The model under review builds one solid part; all positions refer to its coordinate system, in mm. A direction names the side the tool comes from. Coordinates: 2 decimals unless noted, no trailing zeros. Loops run counter-clockwise (first coordinate to the right, second up) from the corner with the lowest first, then second, coordinate; pieces in that order, holes last. Notation, with made-up numbers: (64, 12.25) - (103, 12.25) arc R23 ccw to (103, 46.25) - close; hole circle Ø6 at (12.25, 50.5). An arc over 180 degrees is marked (long way). One line per item, written item: value. Start each with the question number.
1. We need section C-C, the plane y = -8.25. Give the boundary of the cut face in (x, z).
2. We need section D-D, the plane x = -16. Give the boundary of the cut face in (y, z), then the cut area to 3 significant figures.
3. Insertion check: P1, Ø2, axis at y = -11.5, z = 36, coming from the -X side; P2, Ø6, axis at x = 3.5, y = 10, coming from the -Z side; P3, Ø9.5, axis at x = 23, z = 68.5, coming from the -Y side. Each pin has a flat end and moves straight along its axis. Give the tip position at first contact, or say it passes through.
4. For faces 5 (the face through (12.35, -12, 33)), 6 (the face through (21.34, -1.45, 64.78)), 7 (the face through (-25.8, 6, -1)), 8 (the face through (-24.48, 7.84, 64.98)), list the 3-axis set-ups (+Z, -Z, +X, -X, +Y, -Y) from which the entire face can be reached by the end or side of a thin tool; tool diameter is ignored.
5. Mouldability with a two-part tool opening along Y and no side actions: class faces 1 (the face through (-10, -10, 33)), 2 (the face through (-22, 8, 70.025)), 3 (the face through (0, -9, 31.02)), 4 (the face through (-21.5, -1.45, 1.4)) as +Y half, -Y half, draft (parallel to the pull), parting line (faces both ways), or undercut.
6. We need section B-B, the plane z = 43.5. Give the boundary of the cut face in (x, y).
7. To check wall thickness, follow line 1 (Y direction, x = 0, z = 30.9) (3 decimals); line 2 (Z direction, x = 17.5, y = 11.25); line 3 (Y direction, x = 0, z = 59). State the ranges of each line that lie inside material, in increasing order.
8. We need section A-A, the plane x = 21.59. Give the boundary of the cut face in (y, z) (3 decimals).
from build123d import *
from build123d.topology import SkipClean

# Parameters (mm, degrees)
SKETCH1_W                = 34
SKETCH1_H                = 28.5
BOSS_EXTRUDE1_DEPTH      = 66.04
SKETCH3_R                = 12.35
CUT_EXTRUDE1_DEPTH       = 70.665946488
SKETCH7_W                = 8.8
SKETCH7_H                = 15.7
BOSS_EXTRUDE2_DEPTH      = 4.93
BOSS_EXTRUDE2_DEPTH_BACK = 3.72
SKETCH10_W               = 8.8
SKETCH10_H               = 15.7
BOSS_EXTRUDE3_DEPTH      = 3.72
BOSS_EXTRUDE3_DEPTH_BACK = 4.93
CUT_EXTRUDE5_DEPTH       = 13
SKETCH11_R               = 12.35
BOSS_EXTRUDE4_DEPTH      = 2
CUT_EXTRUDE7_DEPTH       = 11.43
SKETCH14_R               = 6
BOSS_EXTRUDE5_DEPTH      = 3.1
SKETCH15_R               = 3.325
CUT_EXTRUDE8_DEPTH       = 2.5
SKETCH16_R               = 3.325
CUT_EXTRUDE9_DEPTH       = 2.5
SKETCH25_R               = 1.75
CUT_EXTRUDE17_DEPTH      = 50


with BuildPart() as part:
    # Sketch1 → Boss-Extrude1 (new body)
    with BuildSketch(Plane.XY):
        Rectangle(SKETCH1_W, SKETCH1_H)
    extrude(amount=BOSS_EXTRUDE1_DEPTH)

    # Sketch3 → Cut-Extrude1 (cut, through all)
    with BuildSketch(Plane.XY.offset(66.04)):
        Circle(SKETCH3_R)
    extrude(amount=-CUT_EXTRUDE1_DEPTH, mode=Mode.SUBTRACT)

    # Sketch7 → Boss-Extrude2 (add, two sides)
    with BuildSketch(Plane.XY.offset(66.04)) as boss_extrude2_sk:
        with Locations((-21.4, 6.4)):
            Rectangle(SKETCH7_W, SKETCH7_H)
        with Locations((21.4, 6.4)):
            Rectangle(SKETCH7_W, SKETCH7_H)
    extrude(amount=BOSS_EXTRUDE2_DEPTH)
    extrude(boss_extrude2_sk.sketch, amount=-BOSS_EXTRUDE2_DEPTH_BACK)

    # Sketch10 → Boss-Extrude3 (add, two sides)
    with BuildSketch(Plane.XY) as boss_extrude3_sk:
        with Locations((-21.4, 6.4)):
            Rectangle(SKETCH10_W, SKETCH10_H)
        with Locations((21.4, 6.4)):
            Rectangle(SKETCH10_W, SKETCH10_H)
    extrude(amount=BOSS_EXTRUDE3_DEPTH)
    extrude(boss_extrude3_sk.sketch, amount=-BOSS_EXTRUDE3_DEPTH_BACK)

    # Sketch8 → Cut-Extrude5 (cut)
    with BuildSketch(Plane(origin=(0, 14.25, 0), x_dir=(1, 0, 0), z_dir=(0, 1, 0))):
        Polygon((-25.458246804, 0.635), (-23.524123402, -2.715), (-19.655876598, -2.715), (-17.721753196, 0.635), (-19.655876598, 3.985), (-23.524123402, 3.985), align=None)
        Polygon((-17.721753196, -66.675), (-19.655876598, -63.325), (-23.524123402, -63.325), (-25.458246804, -66.675), (-23.524123402, -70.025), (-19.655876598, -70.025), align=None)
        Polygon((17.721753196, -66.675), (19.655876598, -70.025), (23.524123402, -70.025), (25.458246804, -66.675), (23.524123402, -63.325), (19.655876598, -63.325), align=None)
        Polygon((25.458246804, 0.635), (23.524123402, 3.985), (19.655876598, 3.985), (17.721753196, 0.635), (19.655876598, -2.715), (23.524123402, -2.715), align=None)
    extrude(amount=-CUT_EXTRUDE5_DEPTH, mode=Mode.SUBTRACT)


with BuildPart() as body_2:
    # Sketch11 → Boss-Extrude4 (new, symmetric)
    with BuildSketch(Plane.XY.offset(33.02)):
        Circle(SKETCH11_R)
    extrude(amount=BOSS_EXTRUDE4_DEPTH, both=True)


with BuildPart() as cut_extrude7_tool:
    # Sketch13 → Cut-Extrude7 (new, symmetric)
    with SkipClean():  # the faces are left unmerged after this step: merging them gives an invalid solid
        with BuildSketch(Plane.XY.offset(33.02)):
            with BuildLine():
                Line((17, -14.25), (17, 14.25))
                Line((17, 14.25), (12.35, 14.25))
                Line((12.35, 14.25), (12.35, 10))
                Line((12.35, 10), (7.247240854, 10))
                ThreePointArc((7.247240854, 10), (5.218397556, 11.193338508), (3, 11.980087646))
                Line((3, 11.980087646), (3, 0))
                Line((3, 0), (3, -11.980087646))
                ThreePointArc((3, -11.980087646), (5.218397556, -11.193338508), (7.247240854, -10))
                Line((7.247240854, -10), (12.35, -10))
                Line((12.35, -10), (12.35, -14.25))
                Line((12.35, -14.25), (17, -14.25))
            make_face()
            with BuildLine():
                Line((-12.35, 10), (-7.247240854, 10))
                ThreePointArc((-7.247240854, 10), (-5.218397556, 11.193338508), (-3, 11.980087646))
                Line((-3, 11.980087646), (-3, 0))
                Line((-3, 0), (-3, -11.980087646))
                ThreePointArc((-3, -11.980087646), (-5.218397556, -11.193338508), (-7.247240854, -10))
                Line((-7.247240854, -10), (-12.35, -10))
                Line((-12.35, -10), (-12.35, -14.25))
                Line((-12.35, -14.25), (-17, -14.25))
                Line((-17, -14.25), (-17, 14.25))
                Line((-17, 14.25), (-12.35, 14.25))
                Line((-12.35, 14.25), (-12.35, 10))
            make_face()
        extrude(amount=CUT_EXTRUDE7_DEPTH, both=True)


with BuildPart() as part_1:
    with SkipClean():  # the faces are left unmerged after this step: merging them gives an invalid solid
        add(part.part)

        # Cut-Extrude7: cut by cut_extrude7_tool
        add(cut_extrude7_tool.part, mode=Mode.SUBTRACT)



with BuildPart() as body_2_1:
    with SkipClean():  # the faces are left unmerged after this step: merging them gives an invalid solid
        add(body_2.part)

        # Cut-Extrude7: cut by cut_extrude7_tool
        add(cut_extrude7_tool.part, mode=Mode.SUBTRACT)


with BuildPart() as part_2:
    with SkipClean():  # the faces are left unmerged after this step: merging them gives an invalid solid
        add(part_1.part)

        add(body_2_1.part)  # Boss-Extrude5 merges body 2
        # Sketch14 → Boss-Extrude5 (add, symmetric)
        with BuildSketch(Plane.XY.offset(33.02)):
            Circle(SKETCH14_R)
        extrude(amount=BOSS_EXTRUDE5_DEPTH, both=True)

    # Sketch15 → Cut-Extrude8 (cut)
    with SkipClean():  # the faces are left unmerged after this step: merging them gives an invalid solid
        with BuildSketch(Plane.XY.offset(36.12)):
            Circle(SKETCH15_R)
        extrude(amount=-CUT_EXTRUDE8_DEPTH, mode=Mode.SUBTRACT)

    # Sketch16 → Cut-Extrude9 (cut)
    with SkipClean():  # the faces are left unmerged after this step: merging them gives an invalid solid
        with BuildSketch(Plane(origin=(0, 0, 29.92), x_dir=(-1, 0, 0), z_dir=(0, 0, -1))):
            with Locations(Location((0, 0, 0), (0, 0, 180))):
                Circle(SKETCH16_R)
        extrude(amount=-CUT_EXTRUDE9_DEPTH, mode=Mode.SUBTRACT)

    # Sketch25 → Cut-Extrude17 (cut)
    with SkipClean():  # the faces are left unmerged after this step: merging them gives an invalid solid
        with BuildSketch(Plane(origin=(132.323959999, 1.25, 1.846345109), x_dir=(1, 0, 0), z_dir=(0, 1, 0))):
            with Locations(Location((-110.733959999, 2.481345109, 0), (0, 0, 270))):
                Circle(SKETCH25_R)
            with Locations(Location((-110.733959999, -64.828654891, 0), (0, 0, 270))):
                Circle(SKETCH25_R)
            with Locations(Location((-153.913959999, -64.828654891, 0), (0, 0, 270))):
                Circle(SKETCH25_R)
            with Locations(Location((-153.913959999, 2.481345109, 0), (0, 0, 270))):
                Circle(SKETCH25_R)
        extrude(amount=-CUT_EXTRUDE17_DEPTH, mode=Mode.SUBTRACT)


solid = part_2.part
Findings below:
1. outline: (-17, 0) - (-9.19, 0) - (-9.19, 21.59) - (-17, 21.59) - close; (-17, 44.45) - (-9.19, 44.45) - (-9.19, 66.04) - (-17, 66.04) - close; (-3, 31.02) - (3, 31.02) - (3, 35.02) - (-3, 35.02) - close; (9.19, 0) - (17, 0) - (17, 21.59) - (9.19, 21.59) - close; (9.19, 44.45) - (17, 44.45) - (17, 66.04) - (9.19, 66.04) - close
2. outline: (-14.25, 0) - (14.25, 0) - (14.25, 21.59) - (-14.25, 21.59) - close; (-14.25, 44.45) - (14.25, 44.45) - (14.25, 66.04) - (-14.25, 66.04) - close
2. area: 1,230 mm2
3. P1: x = -12.35
3. P2: z = 0
3. P3: y = -1.45
4. face 5: +X, +Y, -Y
4. face 6: +Z, -Z, +X, -Y
4. face 7: +Z, -Z, -X, +Y, -Y
4. face 8: +Y
5. face 1: undercut
5. face 2: draft
5. face 3: undercut
5. face 4: -Y half
6. outline: (-12.35, -14.25) - (12.35, -14.25) - (12.35, -10) - (7.25, -10) arc R12.35 cw to (-7.25, -10) - (-12.35, -10) - close; (-12.35, 10) - (-7.25, 10) arc R12.35 cw to (7.25, 10) - (12.35, 10) - (12.35, 14.25) - (-12.35, 14.25) - close
7. line 1: -14.25 to -12.35, -6 to -3.325, 3.325 to 6, 12.35 to 14.25
7. line 2: -4.93 to 3.72, 62.32 to 70.97
7. line 3: -14.25 to -12.35, 12.35 to 14.25
8. outline: (-1.45, -4.93) - (14.25, -4.93) - (14.25, -3.985) - (1.25, -3.985) - (1.25, -2.385) - (-1.45, -2.385) - close; (-1.45, 1.115) - (1.25, 1.115) - (1.25, 2.715) - (14.25, 2.715) - (14.25, 3.72) - (-1.45, 3.72) - close; (-1.45, 62.32) - (14.25, 62.32) - (14.25, 63.325) - (1.25, 63.325) - (1.25, 64.925) - (-1.45, 64.925) - close; (-1.45, 68.425) - (1.25, 68.425) - (1.25, 70.025) - (14.25, 70.025) - (14.25, 70.97) - (-1.45, 70.97) - close
